from build123d import *
from build123d.topology import SkipClean

# Parameters (mm, degrees)
ESQUISSE1_R             = 50
BOSS_EXTRU_1_DEPTH      = 22
ESQUISSE2_R             = 2.5
ENL_V_MAT_EXTRU_1_DEPTH = 7
ENL_V_START             = -15
ENL_V_MAT_EXTRU_3_DEPTH = 15
ESQUISSE4_R             = 46.5
ESQUISSE4_R_2           = 6
ENL_V_MAT_EXTRU_4_DEPTH = 8
ENL_V_START_2           = -8
ESQUISSE5_R             = 46.5
ESQUISSE5_R_2           = 6
ENL_V_MAT_EXTRU_5_DEPTH = 8
ESQUISSE6_R             = 10
ENL_V_MAT_EXTRU_6_DEPTH = 8
ESQUISSE7_R             = 10
ENL_V_MAT_EXTRU_7_DEPTH = 8
ESQUISSE8_R             = 10
ENL_V_MAT_EXTRU_8_DEPTH = 8
ESQUISSE9_R             = 10
ENL_V_MAT_EXTRU_9_DEPTH = 8


with BuildPart() as part:
    # Esquisse1 → Boss.-Extru.1 (new body)
    with BuildSketch(Plane(origin=(0, 0, 0), x_dir=(1, 0, 0), z_dir=(0, 1, 0))):
        with Locations(Location((0, 0, 0), (0, 0, 270))):
            Circle(ESQUISSE1_R)
    extrude(amount=BOSS_EXTRU_1_DEPTH)

    # Esquisse2 → Enlèv. mat.-Extru.1 (cut)
    with BuildSketch(Plane(origin=(0, 22, 0), x_dir=(1, 0, 0), z_dir=(0, 1, 0))):
        with Locations(Location((0, 0, 0), (0, 0, 270))):
            Circle(ESQUISSE2_R)
    extrude(amount=-ENL_V_MAT_EXTRU_1_DEPTH, mode=Mode.SUBTRACT)

    # Esquisse3 → Enlèv. mat.-Extru.3 (cut)
    with SkipClean():  # the faces are left unmerged after this step: merging them gives an invalid solid
        with BuildSketch(Plane(origin=(0, 0, 0), x_dir=(-1, 0, 0), z_dir=(0, -1, 0)).offset(ENL_V_START)):
            with BuildLine():
                ThreePointArc((2.415699998, 0.643734045), (-2.479075587, 0.322775824), (2.170328924, -1.240835348))
                Line((2.170328924, -1.240835348), (2.415699998, 0.643734045))
            make_face()
        extrude(amount=ENL_V_MAT_EXTRU_3_DEPTH, mode=Mode.SUBTRACT)

    # Esquisse4 → Enlèv. mat.-Extru.4 (cut)
    with SkipClean():  # the faces are left unmerged after this step: merging them gives an invalid solid
        with BuildSketch(Plane(origin=(0, 22, 0), x_dir=(1, 0, 0), z_dir=(0, 1, 0))):
            with Locations(Location((0, 0, 0), (0, 0, 270))):
                Circle(ESQUISSE4_R)
            with Locations(Location((0, 0, 0), (0, 0, 270))):
                Circle(ESQUISSE4_R_2, mode=Mode.SUBTRACT)
        extrude(amount=-ENL_V_MAT_EXTRU_4_DEPTH, mode=Mode.SUBTRACT)

    # Esquisse5 → Enlèv. mat.-Extru.5 (cut)
    with SkipClean():  # the faces are left unmerged after this step: merging them gives an invalid solid
        with BuildSketch(Plane(origin=(0, 0, 0), x_dir=(-1, 0, 0), z_dir=(0, -1, 0)).offset(ENL_V_START_2)):
            with Locations(Location((0, 0, 0), (0, 0, 270))):
                Circle(ESQUISSE5_R)
            with Locations(Location((0, 0, 0), (0, 0, 270))):
                Circle(ESQUISSE5_R_2, mode=Mode.SUBTRACT)
        extrude(amount=ENL_V_MAT_EXTRU_5_DEPTH, mode=Mode.SUBTRACT)

    # Esquisse6 → Enlèv. mat.-Extru.6 (cut)
    with SkipClean():  # the faces are left unmerged after this step: merging them gives an invalid solid
        with BuildSketch(Plane(origin=(0, 14, 0), x_dir=(1, 0, 0), z_dir=(0, 1, 0))):
            with Locations(Location((0, 25, 0), (0, 0, 270))):
                Circle(ESQUISSE6_R)
        extrude(amount=-ENL_V_MAT_EXTRU_6_DEPTH, mode=Mode.SUBTRACT)

    # Esquisse7 → Enlèv. mat.-Extru.7 (cut)
    with SkipClean():  # the faces are left unmerged after this step: merging them gives an invalid solid
        with BuildSketch(Plane(origin=(0, 14, 0), x_dir=(1, 0, 0), z_dir=(0, 1, 0))):
            with Locations(Location((25, 0, 0), (0, 0, 270))):
                Circle(ESQUISSE7_R)
        extrude(amount=-ENL_V_MAT_EXTRU_7_DEPTH, mode=Mode.SUBTRACT)

    # Esquisse8 → Enlèv. mat.-Extru.8 (cut)
    with SkipClean():  # the faces are left unmerged after this step: merging them gives an invalid solid
        with BuildSketch(Plane(origin=(0, 14, 0), x_dir=(1, 0, 0), z_dir=(0, 1, 0))):
            with Locations(Location((0, -25, 0), (0, 0, 270))):
                Circle(ESQUISSE8_R)
        extrude(amount=-ENL_V_MAT_EXTRU_8_DEPTH, mode=Mode.SUBTRACT)

    # Esquisse9 → Enlèv. mat.-Extru.9 (cut)
    with SkipClean():  # the faces are left unmerged after this step: merging them gives an invalid solid
        with BuildSketch(Plane(origin=(0, 14, 0), x_dir=(1, 0, 0), z_dir=(0, 1, 0))):
            with Locations(Location((-25, 0, 0), (0, 0, 270))):
                Circle(ESQUISSE9_R)
        extrude(amount=-ENL_V_MAT_EXTRU_9_DEPTH, mode=Mode.SUBTRACT)


solid = part.part
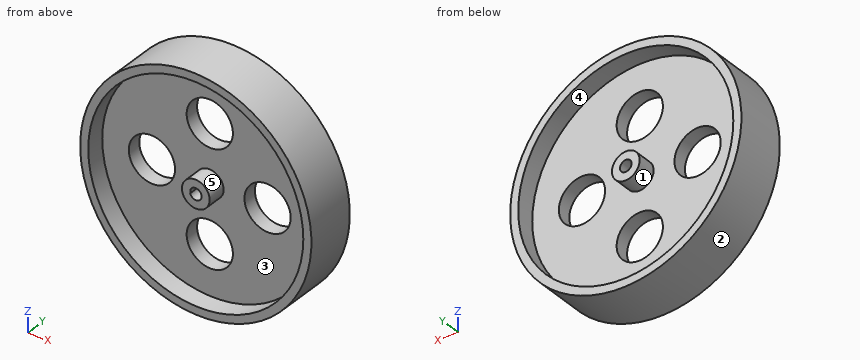
Model file for the job. Use its own axes, mm. Face numbers are marked on the shaded views. A direction names the side the tool comes from. Give positions to 0.01 mm unless a question says otherwise; leave off trailing zeros. Loops run counter-clockwise (first coordinate to the right, second up) from the corner with the lowest first, then second, coordinate; pieces in that order, holes last.
1) Wall check: line 1 (X direction, y = 11.9, z = 0); line 2 (Y direction, x = 12.5, z = -35.5); line 3 (Z direction, x = 19, y = 7). Give the ranges that are in metal, low to high.
2) Pull direction Z, two halves, no side cores. Call the marked faces 1, 2 and 3: +Z half, -Z half, draft (parallel to the pull), parting line (faces both ways), or undercut.
3) Saw through at C-C (x = 27). Write the cut outline in (y, z).
4) Tool access for the marked faces 4 and 5: list every direction of +Z, -Z, +X, -X, +Y, -Y with a clear straight run to the whole face (end or side of a thin tool).
5) Saw through at B-B (y = 4.25). Write the cut outline in (x, z).
6) Saw through at D-D (z = -25). Write the cut outline in (x, y), plus the area to 3 significant figures.
7) Saw through at A-A (x = 0). Count the separate pieces of the cut face and the enclosed holes in it, plus the area to 3 significant figures.
8) Flat gauge pins, fed straight in: pin 1 Ø18 at (x, z) = (25, 0) entering from +Y; pin 2 Ø12 at (x, z) = (-15.5, 39.5) entering from +Y; pin 3 Ø5 at (x, z) = (27.5, 18.5) entering from +Y; pin 4 Ø5 at (x, y) = (-33, 4) entering from +Z. Where does each tip first touch, or does it go through?
Answer block:
1. line 1: x = -50 to -35, -15 to -2.33, 2.5 to 15, 35 to 50
1. line 2: y = 8 to 14
1. line 3: z = -46.25 to -42.44, 42.44 to 46.25
2. face 1: undercut
2. face 2: parting line
2. face 3: undercut
3. outline: (0, -42.08) - (22, -42.08) - (22, -37.86) - (14, -37.86) - (14, -9.8) - (8, -9.8) - (8, -37.86) - (0, -37.86) - close; (0, 37.86) - (8, 37.86) - (8, 9.8) - (14, 9.8) - (14, 37.86) - (22, 37.86) - (22, 42.08) - (0, 42.08) - close
4. face 4: +Y
4. face 5: -Y
5. outline: circle Ø100 at (0, 0); circle Ø12 at (0, 0); hole circle Ø93 at (0, 0); hole (-2.42, -0.64) arc R2.5 ccw (long way) to (-2.17, 1.24) - close
6. outline: (-43.3, 0) - (-39.21, 0) - (-39.21, 8) - (-10, 8) - (-10, 14) - (-39.21, 14) - (-39.21, 22) - (-43.3, 22) - close; (10, 8) - (39.21, 8) - (39.21, 0) - (43.3, 0) - (43.3, 22) - (39.21, 22) - (39.21, 14) - (10, 14) - close
6. area: 531 mm2
7. separate pieces: 4
7. enclosed holes: 0
7. area: 554 mm2
8. pin 1: passes through
8. pin 2: stops at y = 22
8. pin 3: stops at y = 14
8. pin 4: stops at z = 39.62
